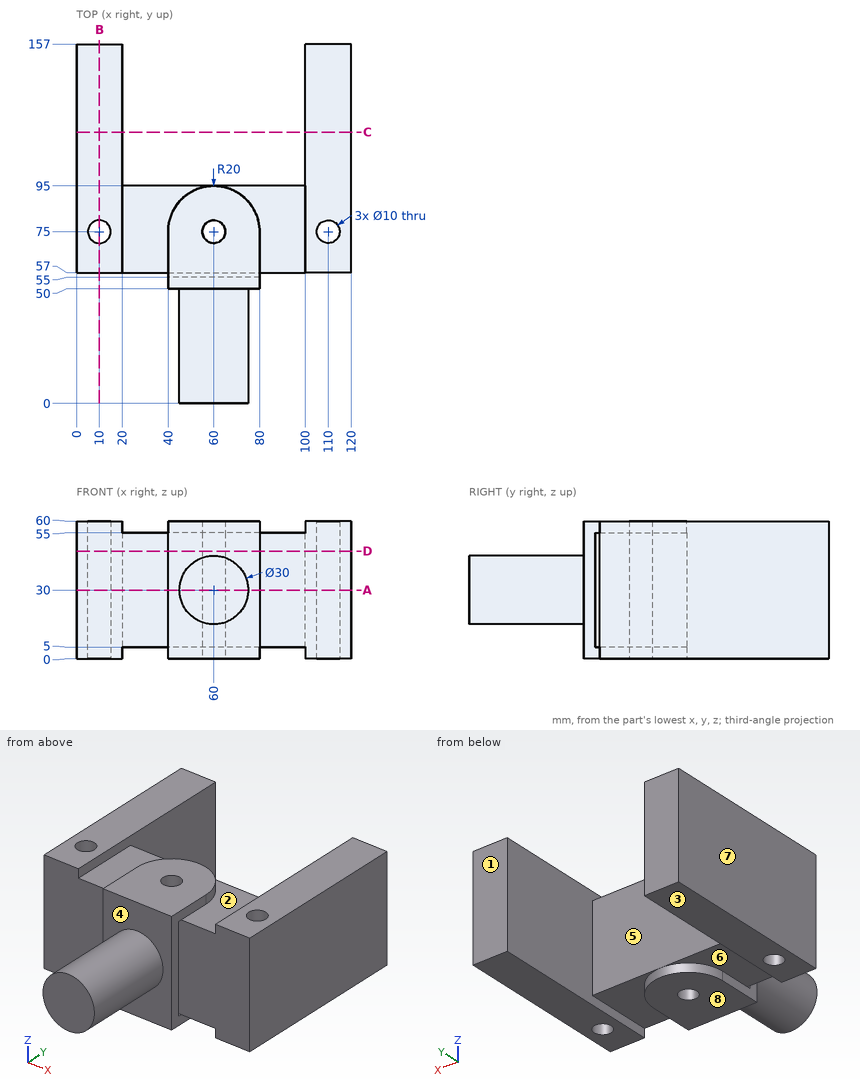
For this review, use the dimensioned drawing (mm, ordinates from the lowest corner) and the shaded views. A direction names the side the tool comes from. Round coordinates to 2 decimals unless told otherwise and drop trailing zeros. Order: outer loops, then holes, each group sorted by start corner. A loop starts at its lowest first (then second) coordinate and runs counter-clockwise, first axis right, second up. Notation, with made-up numbers: M -21,45.25 L -13,45.25 A31 ccw -13,78.25 Z; hole C 86,59.25 d2. An arc over 180 degrees is marked long. Use a Markdown table: item, result. Add a question column.
Item 1: Add section B-B, the plane x = 10. Give the boundary of the cut face in (y, z), then the cut area to 3 significant figures.
Item 2: Insertion check: pin 1 (1.5 mm diameter, centred on x = 84.5, z = 20.5, fed in from -Y); pin 2 (1 mm diameter, centred on x = 80, z = 16, fed in from +Y); pin 3 (5 mm diameter, centred on y = 26.5, z = 22, fed in from +X). Each pin has a flat end and moves straight along its axis. Give the tip position at first contact, or say it passes through.
Item 3: Mouldability with a two-part tool opening along X and no side actions: class the marked faces 6, 7 and 8 as released by +X, released by -X, zero draft, split by the parting line, or undercut.
Item 4: Add section A-A, the plane z = 30. Give the boundary of the cut face in (x, y).
Item 5: To check wall thickness, follow line 1 along Y through (x, z) = (60, 31); line 2 along Y through (x, z) = (110, 47); line 3 along Y through (x, z) = (66.5, 23.5). State the ranges of each line that lie inside material, in increasing order.
Item 6: Add section D-D, the plane z = 47. Give the boundary of the cut face in (x, y).
Item 7: Tool access review of the marked faces 1, 2, 3, 4 and 5: name each direction out of +Z, -Z, +X, -X, +Y, -Y from which nothing blocks a thin tool from reaching the whole face with its end or side.
Item 8: Add section C-C, the plane y = 118.5. Give the boundary of the cut face in (x, z).
Geometry results:
| question | item | result |
|---|---|---|
| 1 | outline | M 57,0 L 70,0 L 70,60 L 57,60 Z; M 80,0 L 157,0 L 157,60 L 80,60 Z |
| 1 | area | 5,400 mm² |
| 2 | pin 1 | stops at y = 57 |
| 2 | pin 2 | stops at y = 95 |
| 2 | pin 3 | stops at x = 73.96 |
| 3 | face 6 | undercut |
| 3 | face 7 | released by -X |
| 3 | face 8 | zero draft |
| 4 | outline | M 0,57 L 120,57 L 120,157 L 100,157 L 100,95 L 20,95 L 20,157 L 0,157 Z; M 40,50 L 45,50 L 45,0 L 75,0 L 75,50 L 80,50 L 80,55 L 40,55 Z; hole C 10,75 d10; hole C 60,75 d10; hole C 110,75 d10 |
| 5 | line 1 | y = 0 to 55, 57 to 70, 80 to 95 |
| 5 | line 2 | y = 57 to 70, 80 to 157 |
| 5 | line 3 | y = 0 to 55, 57 to 95 |
| 6 | outline | M 0,57 L 120,57 L 120,157 L 100,157 L 100,95 L 20,95 L 20,157 L 0,157 Z; M 40,50 L 80,50 L 80,55 L 40,55 Z; hole C 10,75 d10; hole C 60,75 d10; hole C 110,75 d10 |
| 7 | face 1 | +Z, -Z, +X, -X, +Y |
| 7 | face 2 | +Z, +Y |
| 7 | face 3 | -Z, +X, -X, +Y, -Y |
| 7 | face 4 | -Y |
| 7 | face 5 | +Z, -Z, +Y |
| 8 | outline | M 0,0 L 20,0 L 20,60 L 0,60 Z; M 100,0 L 120,0 L 120,60 L 100,60 Z |
